Geometry: final body of the model. Coordinates: model frame, mm. A direction names the side the tool comes from. Give positions to 0.01 mm unless a question says otherwise; leave off trailing zeros. Order: outer loops, then holes, each group sorted by start corner. A loop starts at its lowest first (then second) coordinate and runs counter-clockwise, first axis right, second up. Notation, with made-up numbers: (34.25, 64.25) - (54.25, 64.25) arc R18 cw to (54.25, 85.25) - close; hole circle Ø3 at (0.5, -33). An arc over 180 degrees is marked (long way). Put each result on its own line as item: value. Start each with the question number.
1. First-contact query: P1, Ø1, axis at y = -11, z = -35, coming from the -X side (3 decimals); P2, Ø13.5, axis at y = -11, z = -24, coming from the +X side (3 decimals); P3, Ø7.5, axis at x = 38.5, y = -11.5, coming from the +Z side (3 decimals). Flat tips, straight axial feed; report the tip coordinate or a pass-through.
2. Section C-C on y = -25.5. Return the cut outline in (x, z) (3 decimals).
3. Set-up query: faces 5 (the flat face through (44, -23, 0)), 6 (the flat face through (69, -33.02, 2)), 7 (the flat face through (23, -15.24, -43)). Return all of +Z, -Z, +X, -X, +Y, -Y with unobstructed straight access to the full face (end or side cutting, diameter ignored); none if empty.
4. Ray query, line 1 along X through (y, z) = (-34.5, -42) (3 decimals); line 2 along Z through (x, y) = (2.5, -5) (3 decimals); line 3 along X through (y, z) = (-44, -39) (3 decimals). Return the intervals inside material, ascending. Write a range as from..to.
5. Section B-B on x = 51. Return the cut outline in (y, z) (3 decimals), plus the area to 3 significant figures.
6. Section D-D on z = -25. Return the cut outline in (x, y) (3 decimals).
7. Section A-A on z = -39.37. Return the cut outline in (x, y) (1 decimal), plus the area to 3 significant figures.
8. Mould query, pull axis X, two halves, no side actions, for faces 1 (the flat face through (-13.335, -44, -15)), 2 (the flat face through (102.235, -44, -16)), 3 (the flat face through (45, -44, 13.335)), 4 (the flat face through (67, -2.54, -43)). Classes: pulls with the +X half, pulls with the -X half, needs draft (parallel to the pull), parting line crosses it, or undercut.
from build123d import *

# Parameters (mm, degrees)
SKETCH1_W                = 88.9
SKETCH1_H                = 44.45
BOSS_EXTRUDE1_DEPTH      = 3.175
BOSS_EXTRUDE2_DEPTH      = 45.72
BOSS_EXTRUDE2_DEPTH_BACK = 3.175
SKETCH3_R                = 1.5875
CUT_EXTRUDE1_DEPTH       = 45.72
SKETCH4_W                = 10.16
SKETCH4_H                = 47.625
SKETCH4_H_2              = 10.16
SKETCH4_W_2              = 95.25
BOSS_EXTRUDE3_DEPTH      = 3.175
SKETCH5_R                = 1.5875
CUT_EXTRUDE2_DEPTH       = 3.175
SKETCH6_W                = 20.32
SKETCH6_H                = 11.43
CUT_EXTRUDE3_DEPTH       = 3.175
SKETCH7_W                = 44.45
SKETCH7_H                = 12.7
BOSS_EXTRUDE4_DEPTH      = 3.175


with BuildPart() as part:
    # Sketch1 → Boss-Extrude1 (new body)
    with BuildSketch(Plane(origin=(0, 0, 0), x_dir=(1, 0, 0), z_dir=(0, 1, 0))):
        with Locations((44.45, 22.225)):
            Rectangle(SKETCH1_W, SKETCH1_H)
    extrude(amount=BOSS_EXTRUDE1_DEPTH)

    # Sketch2 → Boss-Extrude2 (add, two sides: drawn at the far end of the back side and taken through both)
    with BuildSketch(Plane.XZ.offset(-BOSS_EXTRUDE2_DEPTH_BACK)):
        Polygon((-3.175, 3.175), (-3.175, -44.45), (0, -44.45), (0, 0), (88.9, 0), (88.9, -44.45), (92.075, -44.45), (92.075, 3.175), align=None)
    extrude(amount=BOSS_EXTRUDE2_DEPTH + BOSS_EXTRUDE2_DEPTH_BACK)

    # Sketch3 → Cut-Extrude1 (cut)
    with BuildSketch(Plane.XZ):
        with Locations(Location((83.34375, -5.588, 0), (0, 0, 270))):
            Circle(SKETCH3_R)
        with Locations(Location((5.55625, -5.588, 0), (0, 0, 270))):
            Circle(SKETCH3_R)
    extrude(amount=-CUT_EXTRUDE1_DEPTH, mode=Mode.SUBTRACT)

    # Sketch4 → Boss-Extrude3 (add)
    with BuildSketch(Plane.XZ.offset(45.72)):
        with Locations((-8.255, -20.6375)):
            Rectangle(SKETCH4_W, SKETCH4_H)
        with Locations((-8.255, 8.255)):
            Rectangle(SKETCH4_W, SKETCH4_H_2)
        with Locations((44.45, 8.255)):
            Rectangle(SKETCH4_W_2, SKETCH4_H_2)
        Polygon((92.075, -44.45), (102.235, -44.45), (102.235, 13.335), (92.075, 13.335), (92.075, 3.175), align=None)
    extrude(amount=-BOSS_EXTRUDE3_DEPTH)

    # Sketch5 → Cut-Extrude2 (cut)
    with BuildSketch(Plane(origin=(0, -42.545, 0), x_dir=(1, 0, 0), z_dir=(0, 1, 0))):
        with Locations(Location((-8.255, 39.37, 0), (0, 0, 270))):
            Circle(SKETCH5_R)
        with Locations(Location((-8.255, -8.255, 0), (0, 0, 270))):
            Circle(SKETCH5_R)
        with Locations(Location((97.155, -8.255, 0), (0, 0, 270))):
            Circle(SKETCH5_R)
        with Locations(Location((97.155, 39.37, 0), (0, 0, 270))):
            Circle(SKETCH5_R)
    extrude(amount=-CUT_EXTRUDE2_DEPTH, mode=Mode.SUBTRACT)

    # Sketch6 → Cut-Extrude3 (cut)
    with BuildSketch(Plane.XY.offset(3.175)):
        with Locations((69.215, -27.305)):
            Rectangle(SKETCH6_W, SKETCH6_H)
    extrude(amount=-CUT_EXTRUDE3_DEPTH, mode=Mode.SUBTRACT)

    # Sketch7 → Boss-Extrude4 (add)
    with BuildSketch(Plane(origin=(0, 0, -44.45), x_dir=(-1, 0, 0), z_dir=(0, 0, -1))):
        with Locations((-22.225, -8.89)):
            Rectangle(SKETCH7_W, SKETCH7_H)
        Polygon((-88.9, 0), (-88.9, -2.54), (-44.45, -2.54), (0, -2.54), (0, 0), align=None)
    extrude(amount=-BOSS_EXTRUDE4_DEPTH)


solid = part.part
Resolved:
1. P1: x = -3.175
1. P2: x = 92.075
1. P3: z = 3.175
2. outline: (-3.175, -44.45) - (0, -44.45) - (0, 0) - (59.055, 0) - (59.055, 3.175) - (-3.175, 3.175) - close; (79.375, 0) - (88.9, 0) - (88.9, -44.45) - (92.075, -44.45) - (92.075, 3.175) - (79.375, 3.175) - close
3. face 5: -Y
3. face 6: +Z, -Z
3. face 7: -Z, -Y
4. line 1: -3.175..0, 88.9..92.075
4. line 2: -44.45..-41.275, 0..3.175
4. line 3: -13.335..-9.799, -6.711..0, 88.9..95.611, 98.699..102.235
5. outline: (-45.72, 0) - (0, 0) - (0, -41.275) - (-2.54, -41.275) - (-2.54, -44.45) - (3.175, -44.45) - (3.175, 3.175) - (-42.545, 3.175) - (-42.545, 13.335) - (-45.72, 13.335) - close
5. area: 337 mm^2
6. outline: (-13.335, -45.72) - (0, -45.72) - (0, 0) - (88.9, 0) - (88.9, -45.72) - (102.235, -45.72) - (102.235, -42.545) - (92.075, -42.545) - (92.075, 3.175) - (-3.175, 3.175) - (-3.175, -42.545) - (-13.335, -42.545) - close
7. outline: (-13.3, -45.7) - (-9.8, -45.7) - (-9.8, -42.5) - (-13.3, -42.5) - close; (-6.7, -45.7) - (0, -45.7) - (0, 0) - (88.9, 0) - (88.9, -45.7) - (95.6, -45.7) - (95.6, -42.5) - (92.1, -42.5) - (92.1, 3.2) - (-3.2, 3.2) - (-3.2, -42.5) - (-6.7, -42.5) - close; (98.7, -45.7) - (102.2, -45.7) - (102.2, -42.5) - (98.7, -42.5) - close
7. area: 637 mm^2
8. face 1: pulls with the -X half
8. face 2: pulls with the +X half
8. face 3: needs draft
8. face 4: undercut
